Could you check a few things on this model? Use its own coordinates, in mm. A direction names the side the tool comes from. Round coordinates to 2 decimals unless told otherwise and drop trailing zeros. Loops run counter-clockwise (first coordinate to the right, second up) from the corner with the lowest first, then second, coordinate; pieces in that order, holes last. Notation, with made-up numbers: (-20, 8) - (-4, 8) arc R31 ccw to (-4, 47) - close; hole circle Ø4 at (3.5, -35.5). An arc over 180 degrees is marked (long way). Use one line per item in the form item = value.
```python
from build123d import *

# Parameters (mm, degrees)
F0_R     = 18.034
F1_DEPTH = 49.911
F3_DEPTH = 11.811
F5_DEPTH = 14.224


with BuildPart() as f1:
    # F0 (on Front) → F1 (new body)
    with BuildSketch(Plane.XZ):
        Circle(F0_R)
    extrude(amount=-F1_DEPTH)

    # F2 (on Front) → F3 (join)
    with BuildSketch(Plane.XZ):
        with BuildLine():
            ThreePointArc((-9.525, 15.3133775177), (0, 18.034), (9.525, 15.3133775177))
            Line((9.525, 15.3133775177), (9.525, 23.2722085544))
            ThreePointArc((9.525, 23.2722085544), (4.8537799544, 24.6731055231), (0, 25.146))
            ThreePointArc((0, 25.146), (-4.8537799544, 24.6731055231), (-9.525, 23.2722085544))
            Line((-9.525, 23.2722085544), (-9.525, 15.3133775177))
        make_face()
    extrude(amount=-F3_DEPTH)

    # F4 (on face) → F5 (join)
    with BuildSketch(Plane(origin=(0, 49.911, 0), x_dir=(-1, 0, 0), z_dir=(0, 1, 0))):
        with BuildLine():
            Line((1.0317528774, 1.2065), (-1.0317528774, 1.2065))
            ThreePointArc((-1.0317528774, 1.2065), (0, -1.5875), (1.0317528774, 1.2065))
        make_face()
    extrude(amount=F5_DEPTH)


solid = f1.part
```
1. If we section it at C-C, the plane x = -7: Write out the boundary of the cut face in (y, z).
Solution:
outline = (0, -16.62) - (49.91, -16.62) - (49.91, 16.62) - (11.81, 16.62) - (11.81, 24.15) - (0, 24.15) - close
2. Please list where these lines run through material, in increasing order: line 1 along Y through (x, z) = (-11.5, -2); line 2 along Z through (x, y) = (-0.5, 18.5); line 3 along Z through (x, y) = (-6, 40).
Solution:
line_1 = 0 to 49.91
line_2 = -18.03 to 18.03
line_3 = -17.01 to 17.01
3. If we section it at B-B, the plane y = 7.5: Write out the boundary of the cut face in (x, z) (3 decimals), plus the area to 3 significant figures.
Solution:
outline = (-9.525, 15.313) arc R18.034 ccw (long way) to (9.525, 15.313) - (9.525, 23.272) arc R25.146 ccw to (-9.525, 23.272) - close
area = 1,160 mm^2
4. On a 3-axis mill with a long thin cutter (end or side, diameter ignored), from which of +Z, -Z, +X, -X, +Y, -Y can I reach the whole of each face in a straight line? I mean faces 1 (the face through (9.525, 6, 19)), 2 (the face through (-9.525, 6, 19)), 3 (the face through (0.054, 56.923, -1.587)), 4 (the face through (0, 64.135, 0)), 5 (the face through (0, 57, 1.206)). Say none if no direction works.
Solution:
face_1 = +Z, +X, +Y, -Y
face_2 = +Z, -X, +Y, -Y
face_3 = +Y
face_4 = +Z, -Z, +X, -X, +Y
face_5 = +Z, +X, -X, +Y
5. If we section it at A-A, the plane z = 0: Write out the boundary of the cut face in (x, y) (1 decimal).
Solution:
outline = (-18, 0) - (18, 0) - (18, 49.9) - (1.6, 49.9) - (1.6, 64.1) - (-1.6, 64.1) - (-1.6, 49.9) - (-18, 49.9) - close
6. If we section it at D-D, the plane x = 6: Write out the boundary of the cut face in (y, z).
Solution:
outline = (0, -17.01) - (49.91, -17.01) - (49.91, 17.01) - (11.81, 17.01) - (11.81, 24.42) - (0, 24.42) - close
7. For P1, Ø12, axis at x = -9.5, y = 7.5, coming from the -Z side; P2, Ø12, axis at x = -4, y = 21.5, coming from the +Z side; P3, Ø10, axis at x = -1.5, y = 57, coming from the +Z side, each with a flat end and sliding along its axis, tell me the tip position at first contact or that it passes through.
Solution:
P1 = -17.69
P2 = 18.03
P3 = 1.21
